Autodesk Inventor part; units mm, degrees
ref_plane "YZ Plane" through (0, 0, 0) normal (1, 0, 0) x (0, 1, 0)
ref_plane "XZ Plane" through (0, 0, 0) normal (0, 1, 0) x (-1, 0, 0)
ref_plane "XY Plane" through (0, 0, 0) normal (0, 0, 1) x (1, 0, 0)
sketch "Sketch1" plane through (0, 0, 0) normal (0, 1, 0) x (-1, 0, 0)
  line L0 (6, -3.4641) -> (0, -6.9282)
  line L1 (0, -6.9282) -> (-6, -3.4641)
  line L2 (-6, -3.4641) -> (-6, 3.4641)
  line L3 (-6, 3.4641) -> (0, 6.9282)
  line L4 (0, 6.9282) -> (6, 3.4641)
  line L5 (6, 3.4641) -> (6, -3.4641)
  circle A0 centre (0, 0) radius 2
  dimension "d0" = 6
  dimension "d1" = 4
extrude "Extrusion1" add sketch "Sketch1" along normal blind 6
sketch "Sketch2" plane through (0, 6, 0) normal (0, 1, 0) x (1, 0, 0)
  circle A0 centre (0, 0) radius 3
  circle A1 centre (0, 0) radius 5.5
  dimension "d4" = 6
  dimension "d5" = 11
extrude "Extrusion2" add sketch "Sketch2" along normal blind 24
sketch "Sketch3" plane through (0, 0, 0) normal (0, 0, 1) x (1, 0, 0)
  circle A0 centre (0, 25) radius 1.5
  line L0 (-5.3, 30) -> (5.3, 30)
  point P0 (0, 0)
  dimension "d16" = 3
extrude "Extrusion3" cut sketch "Sketch3" along normal mid plane 24
chamfer "Chamfer" distance 0.5 angle 45 4 edges at (2, 0, 0) (-3, 30, 0) (-1.5, 25.0054, -5.2915) (-1.5, 25.0054, 5.2915)
sketch "Sketch4" plane through (0, 0, 0) normal (1, 0, 0) x (0, 1, 0)
  line L0 (0, -3.4641) -> (0, -6.9282)
  line L1 (0, -6.9282) -> (0, -5.9282)
  line L2 (0, -6.9282) -> (1, -6.9282)
  line L3 (1, -6.9282) -> (0, -5.9282)
  line L4 (-6, 0) -> (36, 0)
  line L5 (0, -6.9282) -> (6, -6.9282)
  line L6 (6, -6.9282) -> (5, -6.9282)
  line L7 (6, -6.9282) -> (6, -5.9282)
  line L8 (6, -5.9282) -> (5, -6.9282)
  dimension "d31" = 1
  dimension "d32" = 1
  dimension "d36" = 1
  dimension "d37" = 1
revolve "Revolution" cut sketch "Sketch4" angle 360 about axis through (0, -10, 0) along (0, 1, 0)
thread "Thread1"
thread "Thread2"
thread "Thread3"
properties part number "6mmID_30mmL_hex_adapter"
Verification items for the finished model (mm, model axes). A direction names the side the tool comes from. Give positions to 0.01 mm unless a question says otherwise; leave off trailing zeros. Loops run counter-clockwise (first coordinate to the right, second up) from the corner with the lowest first, then second, coordinate; pieces in that order, holes last.
1) Set-up check for faces 1 (the flat face through (-6, 3, 0)), 2 (the cylindrical face through (0, 18, 3)): record each of +Z, -Z, +X, -X, +Y, -Y from which the full face is reachable in a straight line by a thin tool's end or side.
2) Sectioned sample at D-D, the plane y = 14.5. Enter the section's corners in (x, z), then the cut area to 3 significant figures.
3) Depth check by flat-ended pin: pin 1 Ø6.5 at (x, z) = (0, 0) entering from +Y; pin 2 Ø8 at (y, z) = (21, -0.5) entering from -X; pin 3 Ø2.5 at (x, y) = (0, 25) entering from +Z; pin 4 Ø1 at (x, y) = (3, 23) entering from -Z. Enter the tip coordinate at first touch or a pass-through.
4) Thickness scan on line 1 along X through (y, z) = (20, 0); line 2 along Y through (x, z) = (0, 3.7); line 3 along Z through (x, y) = (-2, 23). Record the ranges inside material, lowest first.
5) Sectioned sample at C-C, the plane x = 0.5. Count the separate pieces of the cut face and the enclosed holes in it, then the cut area to 3 significant figures.
6) Draft check along Y on faces 3 (the flat face through (-3, 0, 0)), 4 (the flat face through (-3.042, 2.959, -5.172)), 5 (the cylindrical face through (1.43, 25.45, -3.78)), 6 (the cylindrical face through (1.43, 24.55, 3.78)). Enter one of: pulls with the +Y half, pulls with the -Y half, needs draft (parallel to the pull), parting line crosses it, or undercut.
7) Sectioned sample at B-B, the plane z = 0. Enter the section's corners in (x, y), then the cut area to 3 significant figures.
8) Sectioned sample at A-A, the plane y = 4. Enter the section's corners in (x, z), then the cut area to 3 significant figures.
Answers:
1. face 1: +Z, -Z, -X, +Y, -Y
1. face 2: +Y
2. outline: circle Ø11 at (0, 0); hole circle Ø6 at (0, 0)
2. area: 66.8 mm2
3. pin 1: stops at y = 29.75
3. pin 2: stops at x = -5.5
3. pin 3: passes through
3. pin 4: stops at z = -4.9
4. line 1: x = -5.5 to -3, 3 to 5.5
4. line 2: y = 0 to 23.5, 26.5 to 30
4. line 3: z = -5.12 to -2.24, 2.24 to 5.12
5. separate pieces: 4
5. enclosed holes: 0
5. area: 161 mm2
6. face 3: pulls with the -Y half
6. face 4: needs draft
6. face 5: undercut
6. face 6: undercut
7. outline: (-6, 0.07) - (-5.93, 0) - (-2.5, 0) - (-2, 0.5) - (-2, 6) - (-3, 6) - (-3, 29.5) - (-3.5, 30) - (-5.5, 30) - (-5.5, 6) - (-5.93, 6) - (-6, 5.93) - close; (2, 0.5) - (2.5, 0) - (5.93, 0) - (6, 0.07) - (6, 5.93) - (5.93, 6) - (5.5, 6) - (5.5, 30) - (3.5, 30) - (3, 29.5) - (3, 6) - (2, 6) - close
7. area: 167 mm2
8. outline: (-6, -3.46) - (0, -6.93) - (6, -3.46) - (6, 3.46) - (0, 6.93) - (-6, 3.46) - close; hole circle Ø4 at (0, 0)
8. area: 112 mm2
